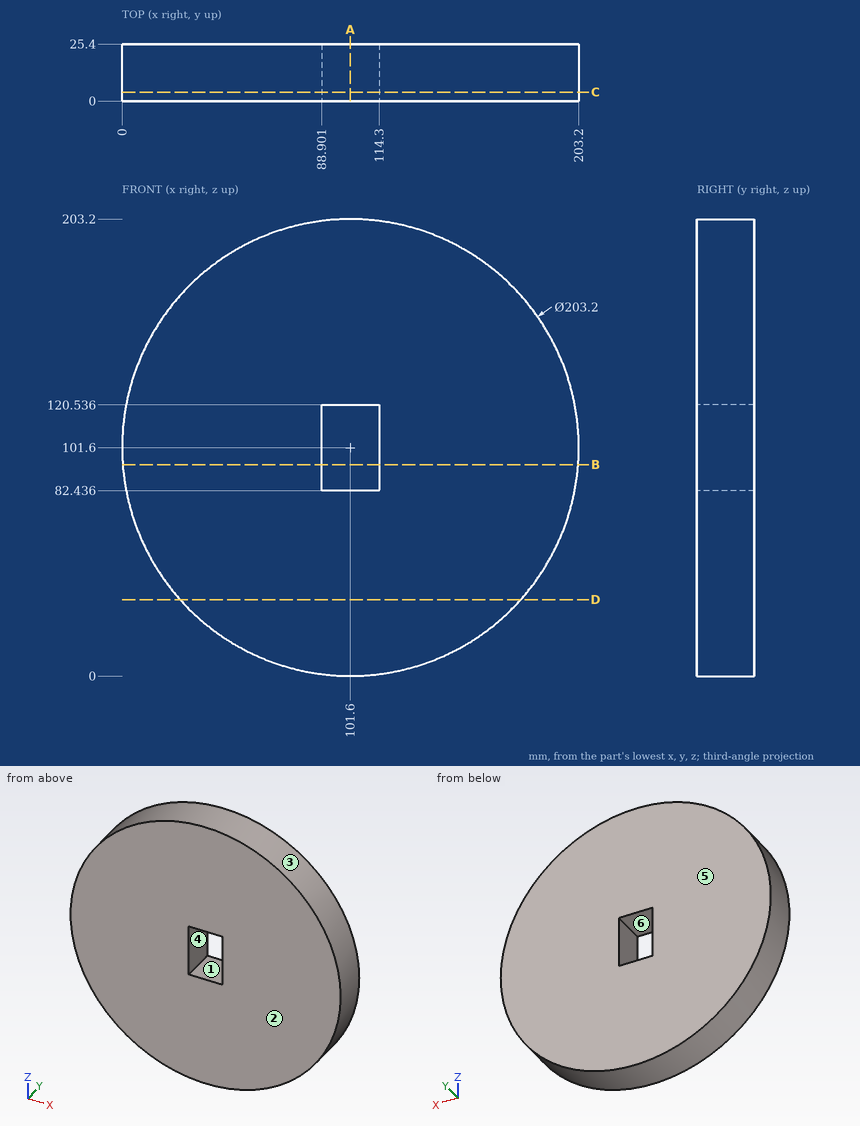
For this review, use the dimensioned drawing (mm, ordinates from the lowest corner) and the shaded views. A direction names the side the tool comes from. Round coordinates to 2 decimals unless told otherwise and drop trailing zeros. Write each loop counter-clockwise with the first axis right and the second up, starting at its lowest first coordinate (ties: lowest second). Pieces come first, ordered by that corner, then holes. Notation, with made-up numbers: (26, 11) -> (70, 11) arc R22 cw to (70, 18) -> close; hole circle Ø7 at (-29.5, -18.5). An arc over 180 degrees is marked (long way). Use one line per item in the form item = value.
Q1. Consider section C-C (y = 4). State the section outline as (x, z) points, then the cut area to 3 significant figures.
Resolved:
outline = circle Ø203.2 at (101.6, 101.6); hole (88.9, 82.44) -> (114.3, 82.44) -> (114.3, 120.54) -> (88.9, 120.54) -> close
area = 31,500 mm²
Q2. To check wall thickness, follow probe 1 along Z at (x, y) = (104.5, 19.5); probe 2 along X at (y, z) = (1.5, 110); probe 3 along X at (y, z) = (21.5, 114.5). State the ranges of each line that lie inside material, in increasing order. Write a range as from..to.
Resolved:
probe_1 = 0.04..82.44, 120.54..203.16
probe_2 = 0.35..88.9, 114.3..202.85
probe_3 = 0.82..88.9, 114.3..202.38
Q3. The part is to be moulded in two halves that separate along Z. For the marked faces 3, 4, 5 and 6, say which applies: released by +Z, released by -Z, zero draft, split by the parting line, or undercut.
Resolved:
face_3 = split by the parting line
face_4 = undercut
face_5 = zero draft
face_6 = undercut
Q4. Consider section B-B (z = 94). State the section outline as (x, y) points (1 decimal), then the cut area to 3 significant figures.
Resolved:
outline = (0.3, 0) -> (88.9, 0) -> (88.9, 25.4) -> (0.3, 25.4) -> close; (114.3, 0) -> (202.9, 0) -> (202.9, 25.4) -> (114.3, 25.4) -> close
area = 4,500 mm²
Q5. Consider section A-A (x = 101.6). State the section outline as (y, z) points, then the cut area to 3 significant figures.
Resolved:
outline = (0, 0) -> (25.4, 0) -> (25.4, 82.44) -> (0, 82.44) -> close; (0, 120.54) -> (25.4, 120.54) -> (25.4, 203.2) -> (0, 203.2) -> close
area = 4,190 mm²
Q6. Machinability: for the marked faces 1 and 2, which of the approach directions +Z, -Z, +X, -X, +Y, -Y give a long, thin tool a straight path to every point of the face, cutting with its end or side? Answer none if there is none.
Resolved:
face_1 = +Y, -Y
face_2 = +Z, -Z, +X, -X, -Y
Q7. Consider section D-D (z = 34). State the section outline as (x, y) points, then the cut area to 3 significant figures.
Resolved:
outline = (25.75, 0) -> (177.45, 0) -> (177.45, 25.4) -> (25.75, 25.4) -> close
area = 3,850 mm²
Q8. Clearance check with flat-ended pins moving along their axes: pin 1 Ø5 at (y, z) = (15, 84) entering from +X; pin 2 Ø8 at (y, z) = (22, 52) entering from +X; pin 3 Ø8 at (x, y) = (115.5, 11.5) entering from +Z. State where each tip first meets the part, or that it passes through.
Resolved:
pin_1 = 202.07
pin_2 = 192.39
pin_3 = 202.72
